Work out the finished part from the listing and answer in its coordinate system (mm). Face numbers are marked on the shaded views. A direction names the side the tool comes from. Coordinates: 2 decimals unless noted, no trailing zeros. Order: outer loops, then holes, each group sorted by start corner. A loop starts at its lowest first (then second) coordinate and runs counter-clockwise, first axis right, second up. Notation, with made-up numbers: M 86.5,61.25 L 120.5,61.25 A21 cw 120.5,93.25 Z; hole C -32,-32.5 d10. An arc over 180 degrees is marked long. Write item = value, one per line. Start each with the question number.
Q1. Find section B-B on z = 29.5. Give the number of separate pieces and of enclosed holes in the cut face, and give its area (3 significant figures).
Q2. Find section C-C on x = -104.5. Give the vertices of the cut face in (y, z).
Q3. A tool of negligible diameter and unlimited length cuts with its end or side. For the marked faces 1 and 2, from which of +Z, -Z, +X, -X, +Y, -Y can it reach the whole face along a straight path? Write none if from no direction.
Q4. Each of these flat-tipped pins is pushed along its axis until it touches: P1, Ø12, axis at x = 127.5, y = -16, coming from the +Z side; P2, Ø11, axis at y = -14, z = 7, coming from the +X side; P3, Ø2, axis at x = -2, z = 34, coming from the -Y side. Where does it stop, or does it pass through?
Q5. Straight lines are drawn through the part: line 1 along X through (y, z) = (10, 37.5); line 2 along Z through (x, y) = (62, -26.5); line 3 along X through (y, z) = (-45.5, 2). For each, find the intervals that lie inside material, in ascending order.
Q6. Determine the mould class of the marked faces 3 and 4 for opening direction X: released by +X, released by -X, zero draft, split by the parting line, or undercut.
Q7. Find section A-A on y = -13. Give the vertices of the cut face in (x, z), and give its area (3 significant figures).
Q8. Find section D-D on y = -41. Give the vertices of the cut face in (x, z), and give its area (3 significant figures).
```python
from build123d import *

# Parameters (mm, degrees)
SKETCH_1_W             = 40
SKETCH_1_H             = 80
SKETCH_1_W_2           = 460
SKETCH_1_R             = 10
EXTRUDE_1_DEPTH        = 10
EXTRUDE_START          = 10
SKETCH_1_3_W           = 460
SKETCH_1_3_H           = 80
SKETCH_1_3_R           = 10
EXTRUDE_2_DEPTH        = 10
EXTRUDE_START_2        = -10
SKETCH_1_4_R           = 10
EXTRUDE_3_DEPTH        = 50
EXTRUDE_4_DEPTH        = 24
PATTERN_LINEAR_2_COUNT = 5
PATTERN_LINEAR_2_PITCH = 70


with BuildPart() as part:
    # 草图1 → 凸台-拉伸1 (new body)
    # profile 1 of 3: a face of its own
    with BuildSketch(Plane.XY):
        with Locations((-212.403603398, -15.911028094)):
            Rectangle(SKETCH_1_W, SKETCH_1_H)
    # profile 2 of 3: a face of its own
    with BuildSketch(Plane.XY):
        with Locations((37.596396602, -15.911028094)):
            Rectangle(SKETCH_1_W_2, SKETCH_1_H)
        with Locations((-124.723239389, -35.911028094)):
            Circle(SKETCH_1_R, mode=Mode.SUBTRACT)
        with Locations((-54.723239389, -35.911028094)):
            Circle(SKETCH_1_R, mode=Mode.SUBTRACT)
        with Locations((15.276760611, -35.911028094)):
            Circle(SKETCH_1_R, mode=Mode.SUBTRACT)
        with Locations((85.276760611, -35.911028094)):
            Circle(SKETCH_1_R, mode=Mode.SUBTRACT)
        with Locations((155.276760611, -35.911028094)):
            Circle(SKETCH_1_R, mode=Mode.SUBTRACT)
        with Locations((-124.723239389, 4.088971906)):
            Circle(SKETCH_1_R, mode=Mode.SUBTRACT)
        with Locations((-54.723239389, 4.088971906)):
            Circle(SKETCH_1_R, mode=Mode.SUBTRACT)
        with Locations((15.276760611, 4.088971906)):
            Circle(SKETCH_1_R, mode=Mode.SUBTRACT)
        with Locations((85.276760611, 4.088971906)):
            Circle(SKETCH_1_R, mode=Mode.SUBTRACT)
        with Locations((155.276760611, 4.088971906)):
            Circle(SKETCH_1_R, mode=Mode.SUBTRACT)
    # profile 3 of 3: a face of its own
    with BuildSketch(Plane.XY):
        with Locations((287.596396602, -15.911028094)):
            Rectangle(SKETCH_1_W, SKETCH_1_H)
    extrude(amount=-EXTRUDE_1_DEPTH)

    # 草图1<3> → 凸台-拉伸2 (add)
    with BuildSketch(Plane.XY.offset(EXTRUDE_START)):
        with Locations((37.596396602, -15.911028094)):
            Rectangle(SKETCH_1_3_W, SKETCH_1_3_H)
        with Locations((-124.723239389, -35.911028094)):
            Circle(SKETCH_1_3_R, mode=Mode.SUBTRACT)
        with Locations((-54.723239389, -35.911028094)):
            Circle(SKETCH_1_3_R, mode=Mode.SUBTRACT)
        with Locations((15.276760611, -35.911028094)):
            Circle(SKETCH_1_3_R, mode=Mode.SUBTRACT)
        with Locations((85.276760611, -35.911028094)):
            Circle(SKETCH_1_3_R, mode=Mode.SUBTRACT)
        with Locations((155.276760611, -35.911028094)):
            Circle(SKETCH_1_3_R, mode=Mode.SUBTRACT)
        with Locations((-124.723239389, 4.088971906)):
            Circle(SKETCH_1_3_R, mode=Mode.SUBTRACT)
        with Locations((-54.723239389, 4.088971906)):
            Circle(SKETCH_1_3_R, mode=Mode.SUBTRACT)
        with Locations((15.276760611, 4.088971906)):
            Circle(SKETCH_1_3_R, mode=Mode.SUBTRACT)
        with Locations((85.276760611, 4.088971906)):
            Circle(SKETCH_1_3_R, mode=Mode.SUBTRACT)
        with Locations((155.276760611, 4.088971906)):
            Circle(SKETCH_1_3_R, mode=Mode.SUBTRACT)
    extrude(amount=-EXTRUDE_2_DEPTH)

    # 草图1<4> → 凸台-拉伸3 (add)
    with BuildSketch(Plane.XY.offset(EXTRUDE_START_2)):
        with Locations((-124.723239389, -35.911028094)):
            Circle(SKETCH_1_4_R)
        with Locations((-124.723239389, 4.088971906)):
            Circle(SKETCH_1_4_R)
        with Locations((-54.723239389, -35.911028094)):
            Circle(SKETCH_1_4_R)
        with Locations((15.276760611, -35.911028094)):
            Circle(SKETCH_1_4_R)
        with Locations((85.276760611, 4.088971906)):
            Circle(SKETCH_1_4_R)
        with Locations((155.276760611, 4.088971906)):
            Circle(SKETCH_1_4_R)
        with Locations((-54.723239389, 4.088971906)):
            Circle(SKETCH_1_4_R)
        with Locations((15.276760611, 4.088971906)):
            Circle(SKETCH_1_4_R)
        with Locations((85.276760611, -35.911028094)):
            Circle(SKETCH_1_4_R)
        with Locations((155.276760611, -35.911028094)):
            Circle(SKETCH_1_4_R)
    extrude(amount=EXTRUDE_3_DEPTH)

    # 草图2 → 凸台-拉伸4 (add)
    with BuildSketch(Plane.XY.offset(10)):
        Polygon((-70.214292819, 1.512613092), (-84.238622357, 2.9154911), (-84.454570484, 0.756694909), (-70.214292819, -0.667784764), align=None)
        Polygon((-70.214292819, -31.154271424), (-70.214292819, -33.334669281), (-84.238622357, -34.737547289), (-84.454570484, -32.578751098), align=None)
    extrude_4 = extrude(amount=EXTRUDE_4_DEPTH)

    # 阵列(线性)2: 凸台-拉伸4 ×5
    with Locations(*[(i * PATTERN_LINEAR_2_PITCH, 0, 0) for i in range(1, PATTERN_LINEAR_2_COUNT)]):
        add(extrude_4)


solid = part.part
```
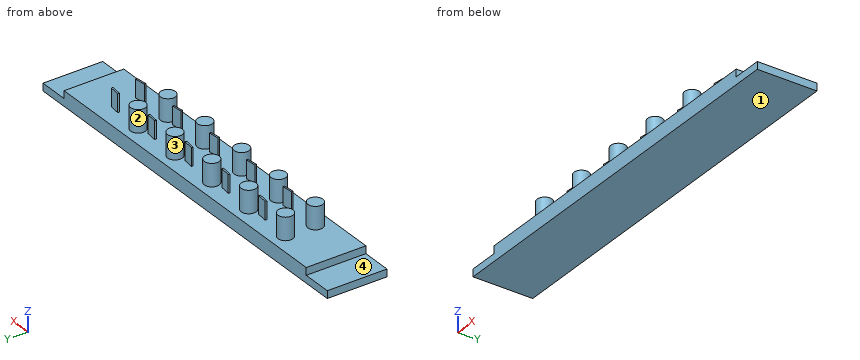
Findings below:
q1.separate_pieces = 20
q1.enclosed_holes = 0
q1.area = 3,450 mm^2
q2.outline = M -55.91,-10 L 24.09,-10 L 24.09,10 L -55.91,10 Z
q3.face_1 = -Z, +X, -X, +Y, -Y
q3.face_2 = +Z
q4.P1 = 10
q4.P2 = 267.6
q4.P3 = -33.61
q5.line_1 = -132.79 to -116.66, -62.79 to -46.66, 7.21 to 23.34, 77.21 to 93.34, 147.21 to 163.34
q5.line_2 = -10 to 10
q5.line_3 = -192.4 to 267.6
q6.face_3 = undercut
q6.face_4 = zero draft
q7.outline = M -232.4,-10 L 307.6,-10 L 307.6,0 L 267.6,0 L 267.6,10 L -192.4,10 L -192.4,0 L -232.4,0 Z
q7.area = 10,000 mm^2
q8.outline = M -232.4,-10 L 307.6,-10 L 307.6,0 L 267.6,0 L 267.6,10 L 163.89,10 L 163.89,40 L 146.67,40 L 146.67,10 L 93.89,10 L 93.89,40 L 76.67,40 L 76.67,10 L 23.89,10 L 23.89,40 L 6.67,40 L 6.67,10 L -46.11,10 L -46.11,40 L -63.33,40 L -63.33,10 L -116.11,10 L -116.11,40 L -133.33,40 L -133.33,10 L -192.4,10 L -192.4,0 L -232.4,0 Z
q8.area = 12,600 mm^2
